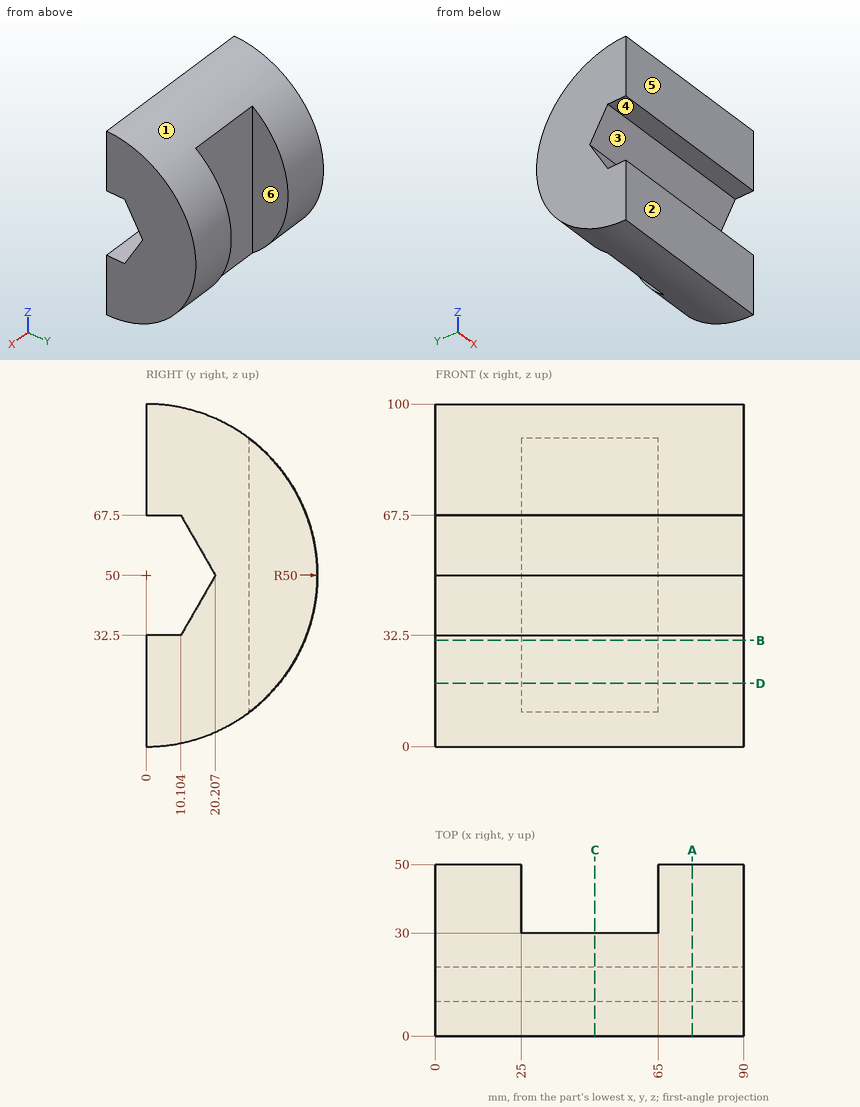
Input: dimensioned drawing with shaded views. Units: mm. Origin: part minimum x, y, z. A direction names the side the tool comes from. Give positions to 0.01 mm unless a question says otherwise; leave off trailing zeros. Loops run counter-clockwise (first coordinate to the right, second up) from the corner with the lowest first, then second, coordinate; pieces in that order, holes last. Notation, with made-up numbers: M 34,-12 L 69,-12 A25 cw 69,9 Z; hole C -20,62 d7. An arc over 180 degrees is marked long. Put each result on its own line as item: value.
1) Reachability of the marked faces 4, 5 and 6 from +Z, -Z, +X, -X, +Y, -Y: full face, straight path, thin tool, end or side. Return the list, or none.
Computed values:
face 4: +X, -X, -Y
face 5: +Z, -Z, +X, -X, -Y
face 6: +Z, -Z, +Y
2) First-contact query: P1, Ø1, axis at x = 22, z = 37.5, coming from the -Y side; P2, Ø20, axis at x = 35.5, z = 63, coming from the +Y side; P3, Ø12, axis at x = 9, y = 14, coming from the +Z side. Flat tips, straight axial feed; report the tip coordinate or a pass-through.
Computed values:
P1: stops at y = 12.7
P2: stops at y = 30
P3: stops at z = 99.36
3) Cut plane D-D, the plane z = 18.5. Return the cut outline in (x, y), plus the area to 3 significant figures.
Computed values:
outline: M 0,0 L 90,0 L 90,38.83 L 65,38.83 L 65,30 L 25,30 L 25,38.83 L 0,38.83 Z
area: 3,140 mm^2
4) Cut plane C-C, the plane x = 46.5. Return the cut outline in (y, z).
Computed values:
outline: M 0,0 A50 ccw 30,10 L 30,90 A50 ccw 0,100 L 0,67.5 L 10.1,67.5 L 20.21,50 L 10.1,32.5 L 0,32.5 Z
5) Cut plane B-B, the plane z = 31. Return the cut outline in (x, y), plus the area to 3 significant figures.
Computed values:
outline: M 0,0 L 90,0 L 90,46.25 L 65,46.25 L 65,30 L 25,30 L 25,46.25 L 0,46.25 Z
area: 3,510 mm^2
6) Cut plane A-A, the plane x = 75. Return the cut outline in (y, z), plus the area to 3 significant figures.
Computed values:
outline: M 0,0 A50 ccw 0,100 L 0,67.5 L 10.1,67.5 L 20.21,50 L 10.1,32.5 L 0,32.5 Z
area: 3,400 mm^2
7) Mould query, pull axis Z, two halves, no side actions, for the marked faces 1, 2 and 3. Classes: released by +Z, released by -Z, zero draft, split by the parting line, or undercut.
Computed values:
face 1: split by the parting line
face 2: zero draft
face 3: undercut
8) Material intervals for L1, parallel to X at y = 38, z = 23; L2, parallel to Y at x = 42.5, z = 29; L3, parallel to Z at x = 82, y = 15 (1 decimal), sorted ascending. Write a range as from..to.
Computed values:
L1: x = 0..25, 65..90
L2: y = 0..30
L3: z = 2.3..41, 59..97.7
